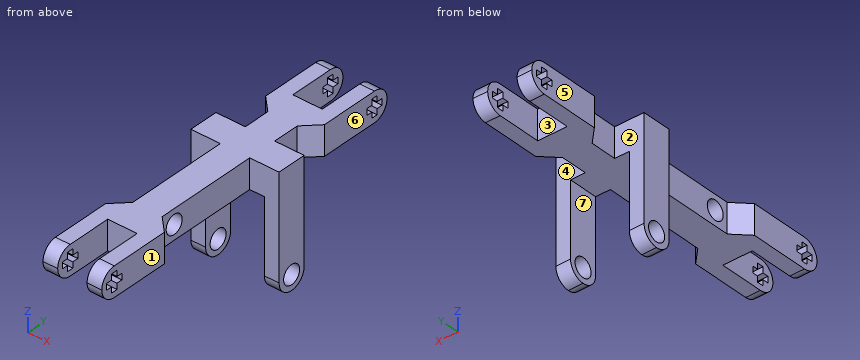
from build123d import *

# Parameters (mm, degrees)
F1_DEPTH  = 7.9375
F2_R      = 2.54
F2_W      = 1.6891
F2_H      = 1.56845
F2_H_2    = 1.6891
F2_W_2    = 1.56845
F3_DEPTH  = 15.875
F4_SIZE   = 3.96874
F5_W      = 7.9375
F5_H      = 7.9375
F6_DEPTH  = 7.9375
F7_W      = 3.96875
F7_H      = 7.9375
F8_DEPTH  = 23.8125
F9_R      = 3.96874
F10_R     = 2.54
F11_DEPTH = 23.8125
F12_W     = 1.6891
F12_H     = 1.56845
F12_W_2   = 1.56845
F12_H_2   = 1.6891
F13_DEPTH = 15.875


# Not quite as in the source:
# - a fillet or chamfer is up to 0.001 mm smaller than in the source, because OpenCascade refuses the exact size


with BuildPart() as f1:
    # F0 (on Top) → F1 (new body)
    with BuildSketch(Plane.XY):
        Polygon((3.96875, 0), (0, 0), (0, -19.84375), (3.96875, -19.84375), (3.96875, -3.96875), (11.90625, -3.96875), (11.90625, -19.84375), (15.875, -19.84375), (15.875, 0), (11.90625, 0), (11.90625, 50.8), (15.875, 50.8), (15.875, 70.64375), (11.90625, 70.64375), (11.90625, 54.76875), (3.96875, 54.76875), (3.96875, 70.64375), (0, 70.64375), (0, 50.8), (3.96875, 50.8), align=None)
    extrude(amount=F1_DEPTH)

    # F2 (on face) → F3 (cut, through all)
    with BuildSketch(Plane.YZ.offset(15.875)):
        with BuildLine():
            ThreePointArc((-15.875, 0), (-18.6813300378, 1.1624199622), (-19.84375, 3.96875))
            Line((-19.84375, 3.96875), (-19.84375, 0))
            Line((-19.84375, 0), (-15.875, 0))
        make_face()
        with BuildLine():
            ThreePointArc((-19.84375, 3.96875), (-18.6813300378, 6.7750800378), (-15.875, 7.9375))
            Line((-15.875, 7.9375), (-19.84375, 7.9375))
            Line((-19.84375, 7.9375), (-19.84375, 3.96875))
        make_face()
        with Locations((7.778559196, 3.96875)):
            Circle(F2_R)
        with Locations((-15.875, 5.597525)):
            Rectangle(F2_W, F2_H)
        with Locations((-15.875, 3.96875)):
            Rectangle(F2_W, F2_H_2)
        with Locations((-17.503775, 3.96875)):
            Rectangle(F2_W_2, F2_H_2)
        with Locations((-14.246225, 3.96875)):
            Rectangle(F2_W_2, F2_H_2)
        with Locations((-15.875, 2.339975)):
            Rectangle(F2_W, F2_H)
    extrude(amount=-F3_DEPTH, mode=Mode.SUBTRACT)

    # F4 (size 3.96875 in the source; OpenCascade refuses exactly that, so slightly less here)
    f4_edges = [f1.edges().sort_by_distance(p)[0] for p in [
        (11.90625, 0, 3.96875),
        (3.96875, 0, 3.96875),
        (11.90625, 50.8, 3.96875),
        (3.96875, 50.8, 3.96875),
    ]]
    chamfer(f4_edges, length=F4_SIZE)

    # F5 (on face) → F6 (join, through all)
    with BuildSketch(Plane.XY.offset(7.9375)):
        with Locations((0, 35.71875)):
            Rectangle(F5_W, F5_H)
        with Locations((15.875, 35.71875)):
            Rectangle(F5_W, F5_H)
    extrude(amount=-F6_DEPTH)

    # F7 (on face) → F8 (join)
    with BuildSketch(Plane(origin=(0, 0, 0), x_dir=(1, 0, 0), z_dir=(0, 0, -1))):
        with Locations((17.859375, -35.71875)):
            Rectangle(F7_W, F7_H)
        with Locations((-1.984375, -35.71875)):
            Rectangle(F7_W, F7_H)
    extrude(amount=F8_DEPTH)

    # F9 (radius 3.96875 in the source; OpenCascade refuses exactly that, so slightly less here)
    f9_edges = [f1.edges().sort_by_distance(p)[0] for p in [
        (-1.984375, 39.6875, -23.8125),
        (-1.984375, 31.75, -23.8125),
        (17.859375, 31.75, -23.8125),
        (17.859375, 39.6875, -23.8125),
        (13.890625, 70.64375, 0),
        (13.890625, 70.64375, 7.9375),
        (1.984375, 70.64375, 7.9375),
        (1.984375, 70.64375, 0),
    ]]
    fillet(f9_edges, radius=F9_R)

    # F10 (on face) → F11 (cut, through all)
    with BuildSketch(Plane(origin=(-3.96875, 0, 0), x_dir=(0, -1, 0), z_dir=(-1, 0, 0))):
        with Locations((-35.71875, -19.84375)):
            Circle(F10_R)
    extrude(amount=-F11_DEPTH, mode=Mode.SUBTRACT)

    # F12 (on face) → F13 (cut, through all)
    with BuildSketch(Plane.YZ.offset(15.875)):
        with Locations((66.675, 2.339975)):
            Rectangle(F12_W, F12_H)
        with Locations((65.046225, 3.96875)):
            Rectangle(F12_W_2, F12_H_2)
        with Locations((66.675, 3.96875)):
            Rectangle(F12_W, F12_H_2)
        with Locations((68.303775, 3.96875)):
            Rectangle(F12_W_2, F12_H_2)
        with Locations((66.675, 5.597525)):
            Rectangle(F12_W, F12_H)
    extrude(amount=-F13_DEPTH, mode=Mode.SUBTRACT)


solid = f1.part
Could you check a few things on this model? Use its own coordinates, in mm. Face numbers are marked on the shaded views. A direction names the side the tool comes from. Give positions to 0.01 mm unless a question says otherwise; leave off trailing zeros. Order: outer loops, then holes, each group sorted by start corner. A loop starts at its lowest first (then second) coordinate and runs counter-clockwise, first axis right, second up. Notation, with made-up numbers: (39.5, -11.5) - (59.5, -11.5) arc R21 ccw to (59.5, 5.5) - close; hole circle Ø8 at (-30.5, -8). An arc over 180 degrees is marked (long way). One line per item, written item: value. Start each with the question number.
1. Thinking about a two-plate mould opening in X: for the marked faces 5, 6 and 7, which applies, +X half, -X half, draft (parallel to the pull), parting line (faces both ways), or undercut?
2. Imagine slicing it at B-B on y = -12.5. List the corners of the cut face in (x, z) for me (1 decimal).
3. For the marked faces 1, 2, 3 and 4, which set-ups out of +Z, -Z, +X, -X, +Y, -Y let a thin tool reach every point of the face, with its end or its side?
4. If I drill on probe 1 along X at (y, z) = (33.5, -13) (3 decimals); probe 2 along Z at (x, y) = (2.75, 65.5); probe 3 along X at (y, z) = (-7.5, 2) (3 decimals), over which ranges is the centre line in solid material (lowest first)?
5. For P1, Ø2, axis at y = 59.5, z = 4.5, coming from the +X side (3 decimals); P2, Ø8, axis at x = 7.5, y = 7.5, coming from the -Z side; P3, Ø6.5, axis at x = -1.5, z = -1, coming from the +Y side, each with a flat end and sliding along its axis, tell me the tip position at first contact or that it passes through.
6. Imagine slicing it at D-D on x = 2.5. Give the number of separate pieces and of enclosed holes in the cut face, plus the area to 3 significant figures.
Values:
1. face 5: -X half
1. face 6: +X half
1. face 7: undercut
2. outline: (0, 0) - (4, 0) - (4, 7.9) - (0, 7.9) - close; (11.9, 0) - (15.9, 0) - (15.9, 7.9) - (11.9, 7.9) - close
3. face 1: +Z, -Z, +X, -Y
3. face 2: +Z, -Z, -X
3. face 3: +Z, -Z, +Y
3. face 4: +Z, -Z, +X
4. probe 1: -3.969 to 0, 15.875 to 19.844
4. probe 2: 0 to 3.12, 4.81 to 7.94
4. probe 3: 0 to 3.969, 11.906 to 15.875
5. P1: x = 15.875
5. P2: z = 0
5. P3: y = 70.05
6. separate pieces: 3
6. enclosed holes: 2
6. area: 377 mm²
